Geometry check sheet. Reference: the model listing, model coordinates, mm. Face numbers are marked on the shaded views. Round coordinates to 2 decimals unless told otherwise and drop trailing zeros. Loops run counter-clockwise (first coordinate to the right, second up) from the corner with the lowest first, then second, coordinate; pieces in that order, holes last. Notation, with made-up numbers: M 57.5,83 L 84.5,83 A15 cw 84.5,106 Z; hole C -28.5,-27 d11. An arc over 180 degrees is marked long. Write item = value, one per line.
from build123d import *

# Parameters (mm, degrees)
F0_R     = 5
F1_DEPTH = 40
F0_R_2   = 8
F2_DEPTH = 3


with BuildPart() as f1:
    # F0 (on Top) → F1 (new body)
    with BuildSketch(Plane.XY):
        with BuildLine():
            ThreePointArc((-3.849529, 5.237473), (-3.941693, 4.313368), (-4.870341, 4.304623))
            ThreePointArc((-4.870341, 4.304623), (-5.077719, 4.057927), (-5.272613, 3.801256))
            ThreePointArc((-5.272613, 3.801256), (-5.076369, 2.893538), (-5.957405, 2.599871))
            ThreePointArc((-5.957405, 2.599871), (-6.078948, 2.301389), (-6.185547, 1.99725))
            ThreePointArc((-6.185547, 1.99725), (-5.719883, 1.193744), (-6.468061, 0.643569))
            ThreePointArc((-6.468061, 0.643569), (-6.49201, 0.32218), (-6.5, 0))
            ThreePointArc((-6.5, 0), (-5.809971, -0.62155), (-6.352903, -1.375002))
            ThreePointArc((-6.352903, -1.375002), (-6.244867, -1.803229), (-6.108002, -2.223131))
            ThreePointArc((-6.108002, -2.223131), (-5.247004, -2.571193), (-5.499497, -3.464899))
            ThreePointArc((-5.499497, -3.464899), (-5.320996, -3.73323), (-5.129413, -3.992383))
            ThreePointArc((-5.129413, -3.992383), (-4.203119, -4.059048), (-4.168789, -4.987103))
            ThreePointArc((-4.168789, -4.987103), (-3.916473, -5.187604), (-3.65453, -5.375352))
            ThreePointArc((-3.65453, -5.375352), (-2.752563, -5.154171), (-2.434731, -6.026781))
            ThreePointArc((-2.434731, -6.026781), (-2.133014, -6.140053), (-1.826053, -6.238231))
            ThreePointArc((-1.826053, -6.238231), (-1.035683, -5.750604), (-0.465101, -6.483339))
            ThreePointArc((-0.465101, -6.483339), (-0.143175, -6.498423), (0.179103, -6.497532))
            ThreePointArc((0.179103, -6.497532), (0.781404, -5.790638), (1.549529, -6.312603))
            ThreePointArc((1.549529, -6.312603), (1.860517, -6.22804), (2.16693, -6.128166))
            ThreePointArc((2.16693, -6.128166), (2.522886, -5.270401), (3.414236, -5.531093))
            ThreePointArc((3.414236, -5.531093), (3.684195, -5.355064), (3.945096, -5.16587))
            ThreePointArc((3.945096, -5.16587), (4.020268, -4.240228), (4.948599, -4.214424))
            ThreePointArc((4.948599, -4.214424), (5.151409, -3.963961), (5.341556, -3.703752))
            ThreePointArc((5.341556, -3.703752), (5.128669, -2.799792), (6.004161, -2.489989))
            ThreePointArc((6.004161, -2.489989), (6.120201, -2.189325), (6.221194, -1.883279))
            ThreePointArc((6.221194, -1.883279), (5.740847, -1.088464), (6.478793, -0.524636))
            ThreePointArc((6.478793, -0.524636), (6.496834, -0.202862), (6.498903, 0.119411))
            ThreePointArc((6.498903, 0.119411), (5.797572, 0.728179), (6.32657, 1.491478))
            ThreePointArc((6.32657, 1.491478), (6.244867, 1.803229), (6.147812, 2.110547))
            ThreePointArc((6.147812, 2.110547), (5.293354, 2.474367), (5.562223, 3.363284))
            ThreePointArc((5.562223, 3.363284), (5.38868, 3.634849), (5.201891, 3.897477))
            ThreePointArc((5.201891, 3.897477), (4.276978, 3.981148), (4.259703, 4.909677))
            ThreePointArc((4.259703, 4.909677), (4.011113, 5.11478), (3.752663, 5.307308))
            ThreePointArc((3.752663, 5.307308), (2.846785, 5.102734), (2.545037, 5.981035))
            ThreePointArc((2.545037, 5.981035), (2.245452, 6.099832), (1.940346, 6.203633))
            ThreePointArc((1.940346, 6.203633), (1.141152, 5.730607), (0.584127, 6.4737))
            ThreePointArc((0.584127, 6.4737), (0.262532, 6.494696), (-0.059708, 6.499726))
            ThreePointArc((-0.059708, 6.499726), (-0.674893, 5.804016), (-1.4333, 6.340004))
            ThreePointArc((-1.4333, 6.340004), (-1.745788, 6.261168), (-2.053985, 6.16694))
            ThreePointArc((-2.053985, 6.16694), (-2.425639, 5.315859), (-3.312049, 5.592882))
            ThreePointArc((-3.312049, 5.592882), (-3.585196, 5.421842), (-3.849529, 5.237473))
        make_face()
        Circle(F0_R, mode=Mode.SUBTRACT)
    extrude(amount=F1_DEPTH)

    # F0 (on Top) → F2 (join)
    with BuildSketch(Plane.XY):
        Circle(F0_R_2)
        with BuildLine():
            ThreePointArc((-5.272613, 3.801256), (-5.077719, 4.057927), (-4.870341, 4.304623))
            ThreePointArc((-4.870341, 4.304623), (-3.941693, 4.313368), (-3.849529, 5.237473))
            ThreePointArc((-3.849529, 5.237473), (-3.585196, 5.421842), (-3.312049, 5.592882))
            ThreePointArc((-3.312049, 5.592882), (-2.425639, 5.315859), (-2.053985, 6.16694))
            ThreePointArc((-2.053985, 6.16694), (-1.745788, 6.261168), (-1.4333, 6.340004))
            ThreePointArc((-1.4333, 6.340004), (-0.674893, 5.804016), (-0.059708, 6.499726))
            ThreePointArc((-0.059708, 6.499726), (0.262532, 6.494696), (0.584127, 6.4737))
            ThreePointArc((0.584127, 6.4737), (1.141152, 5.730607), (1.940346, 6.203633))
            ThreePointArc((1.940346, 6.203633), (2.245452, 6.099832), (2.545037, 5.981035))
            ThreePointArc((2.545037, 5.981035), (2.846785, 5.102734), (3.752663, 5.307308))
            ThreePointArc((3.752663, 5.307308), (4.011113, 5.11478), (4.259703, 4.909677))
            ThreePointArc((4.259703, 4.909677), (4.276978, 3.981148), (5.201891, 3.897477))
            ThreePointArc((5.201891, 3.897477), (5.38868, 3.634849), (5.562223, 3.363284))
            ThreePointArc((5.562223, 3.363284), (5.293354, 2.474367), (6.147812, 2.110547))
            ThreePointArc((6.147812, 2.110547), (6.244867, 1.803229), (6.32657, 1.491478))
            ThreePointArc((6.32657, 1.491478), (5.797572, 0.728179), (6.498903, 0.119411))
            ThreePointArc((6.498903, 0.119411), (6.496834, -0.202862), (6.478793, -0.524636))
            ThreePointArc((6.478793, -0.524636), (5.740847, -1.088464), (6.221194, -1.883279))
            ThreePointArc((6.221194, -1.883279), (6.120201, -2.189325), (6.004161, -2.489989))
            ThreePointArc((6.004161, -2.489989), (5.128669, -2.799792), (5.341556, -3.703752))
            ThreePointArc((5.341556, -3.703752), (5.151409, -3.963961), (4.948599, -4.214424))
            ThreePointArc((4.948599, -4.214424), (4.020268, -4.240228), (3.945096, -5.16587))
            ThreePointArc((3.945096, -5.16587), (3.684195, -5.355064), (3.414236, -5.531093))
            ThreePointArc((3.414236, -5.531093), (2.522886, -5.270401), (2.16693, -6.128166))
            ThreePointArc((2.16693, -6.128166), (1.860517, -6.22804), (1.549529, -6.312603))
            ThreePointArc((1.549529, -6.312603), (0.781404, -5.790638), (0.179103, -6.497532))
            ThreePointArc((0.179103, -6.497532), (-0.143175, -6.498423), (-0.465101, -6.483339))
            ThreePointArc((-0.465101, -6.483339), (-1.035683, -5.750604), (-1.826053, -6.238231))
            ThreePointArc((-1.826053, -6.238231), (-2.133014, -6.140053), (-2.434731, -6.026781))
            ThreePointArc((-2.434731, -6.026781), (-2.752563, -5.154171), (-3.65453, -5.375352))
            ThreePointArc((-3.65453, -5.375352), (-3.916473, -5.187604), (-4.168789, -4.987103))
            ThreePointArc((-4.168789, -4.987103), (-4.203119, -4.059048), (-5.129413, -3.992383))
            ThreePointArc((-5.129413, -3.992383), (-5.320996, -3.73323), (-5.499497, -3.464899))
            ThreePointArc((-5.499497, -3.464899), (-5.247004, -2.571193), (-6.108002, -2.223131))
            ThreePointArc((-6.108002, -2.223131), (-6.244867, -1.803229), (-6.352903, -1.375002))
            ThreePointArc((-6.352903, -1.375002), (-5.809971, -0.62155), (-6.5, 0))
            ThreePointArc((-6.5, 0), (-6.49201, 0.32218), (-6.468061, 0.643569))
            ThreePointArc((-6.468061, 0.643569), (-5.719883, 1.193744), (-6.185547, 1.99725))
            ThreePointArc((-6.185547, 1.99725), (-6.078948, 2.301389), (-5.957405, 2.599871))
            ThreePointArc((-5.957405, 2.599871), (-5.076369, 2.893538), (-5.272613, 3.801256))
        make_face(mode=Mode.SUBTRACT)
    extrude(amount=F2_DEPTH)


solid = f1.part
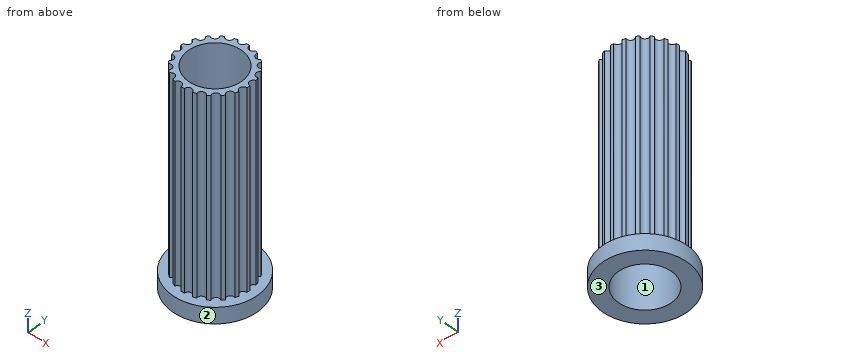
(1) Sectioned sample at A-A on x = -7. Record the cut outline in (y, z), then the cut area to 3 significant figures.
Result set:
outline = M -3.87,0 L 3.87,0 L 3.87,3 L -3.87,3 Z
area = 23.2 mm2
(2) Material ranges on line 1 along Y through (x, z) = (0, 9); line 2 along Y through (x, z) = (-6, 17); line 3 along Z through (x, y) = (-5.75, -5), recorded low to high. Write a range as from..to.
Result set:
line_1 = -6.5..-5, 5..6.5
line_2 = -2.19..-1.18, -0.21..0.77, 1.9..2.5
line_3 = 0..3
(3) Depth check by flat-ended pin: pin 1 Ø1.5 at (y, z) = (1, 25) entering from +X; pin 2 Ø1.5 at (x, z) = (4.5, 34) entering from -Y; pin 3 Ø8 at (x, z) = (-4, 18) entering from +Y. Enter the tip coordinate at first touch or a pass-through.
Result set:
pin_1 = 6.33
pin_2 = -5.31
pin_3 = 6.5
(4) Release check for a two-part mould opening along X. For the marked faces 1, 2 and 3 record: released by +X, released by -X, zero draft, split by the parting line, or undercut.
Result set:
face_1 = undercut
face_2 = split by the parting line
face_3 = zero draft
